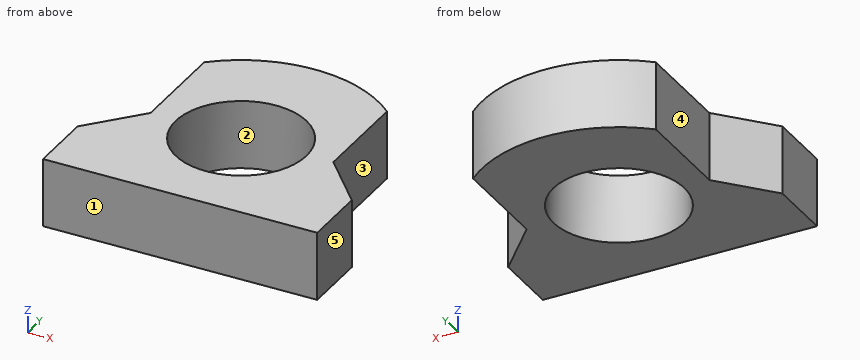
from build123d import *

# Parameters (mm, degrees)
SKETCH1_R           = 14.3
BOSS_EXTRUDE1_DEPTH = 15


with BuildPart() as part:
    # Sketch1 → Boss-Extrude1 (new body)
    with BuildSketch(Plane.XY):
        with BuildLine():
            Line((-30, 0), (30, 0))
            Line((30, 0), (30, 14.180339887))
            Line((30, 14.180339887), (20, 25.360679775))
            Line((20, 25.360679775), (20, 47.360679775))
            ThreePointArc((20, 47.360679775), (0, 55), (-20, 47.360679775))
            Line((-20, 47.360679775), (-20, 25.360679775))
            Line((-20, 25.360679775), (-30, 14.180339887))
            Line((-30, 14.180339887), (-30, 0))
        make_face()
        with Locations((0, 25)):
            Circle(SKETCH1_R, mode=Mode.SUBTRACT)
    extrude(amount=BOSS_EXTRUDE1_DEPTH)


solid = part.part
Read the model definition and answer for the solid it produces. Units are mm, in the model's axes. Face numbers are marked on the shaded views. A direction names the side the tool comes from. Coordinates: 2 decimals unless noted, no trailing zeros. Loops run counter-clockwise (first coordinate to the right, second up) from the corner with the lowest first, then second, coordinate; pieces in that order, holes last. Notation, with made-up numbers: (76.5, 33.25) -> (99.5, 33.25) arc R21 ccw to (99.5, 45.25) -> close; hole circle Ø9 at (-31, 9). An arc over 180 degrees is marked (long way). Write item = value, one per line. Start each with the question number.
1) Given P1, Ø8, axis at y = 41, z = 5.5, coming from the -X side; P2, Ø1, axis at y = 49, z = 13, coming from the +X side; P3, Ø4.5, axis at y = 35, z = 6, coming from the +X side, each flat-ended and moving along its own axis, determine where each tip first touches the part or whether it passes through.
2) The part is cut by section B-B, the plane x = 0. Determine the outline of the cut face in (y, z).
3) Find the intervals of material crossed by L1, parallel to Y at x = 0, z = 8.5; L2, parallel to X at y = 34.5, z = 14.5; L3, parallel to Y at x = 12.5, z = 5.5, in increasing order. Write a range as from..to.
4) The mould has two halves that part along Y. Classify the marked faces 1, 2 and 3: pulls with the +Y half, pulls with the -Y half, needs draft (parallel to the pull), parting line crosses it, or undercut.
5) The part is cut by section A-A, the plane z = 2.25. Determine the outline of the cut face in (x, y).
6) For the marked faces 4 and 5, determine the directions among +Z, -Z, +X, -X, +Y, -Y from which every point of the face is accessible in a straight line to the end or side of a thin tool.
7) The part is cut by section D-D, the plane y = 44.5. Determine the outline of the cut face in (x, z), plus the area to 3 significant figures.
8) The part is cut by section C-C, the plane y = 34.5. Determine the outline of the cut face in (x, z), plus the area to 3 significant figures.
Result:
q1.P1 = -20
q1.P2 = 18.65
q1.P3 = 20
q2.outline = (0, 0) -> (10.7, 0) -> (10.7, 15) -> (0, 15) -> close; (39.3, 0) -> (55, 0) -> (55, 15) -> (39.3, 15) -> close
q3.L1 = 0..10.7, 39.3..55
q3.L2 = -20..-10.69, 10.69..20
q3.L3 = 0..18.05, 31.95..52.27
q4.face_1 = pulls with the -Y half
q4.face_2 = undercut
q4.face_3 = needs draft
q5.outline = (-30, 0) -> (30, 0) -> (30, 14.18) -> (20, 25.36) -> (20, 47.36) arc R30 ccw to (-20, 47.36) -> (-20, 25.36) -> (-30, 14.18) -> close; hole circle Ø28.6 at (0, 25)
q6.face_4 = +Z, -Z, -X, +Y
q6.face_5 = +Z, -Z, +X, +Y, -Y
q7.outline = (-20, 0) -> (20, 0) -> (20, 15) -> (-20, 15) -> close
q7.area = 600 mm²
q8.outline = (-20, 0) -> (-10.69, 0) -> (-10.69, 15) -> (-20, 15) -> close; (10.69, 0) -> (20, 0) -> (20, 15) -> (10.69, 15) -> close
q8.area = 279 mm²
